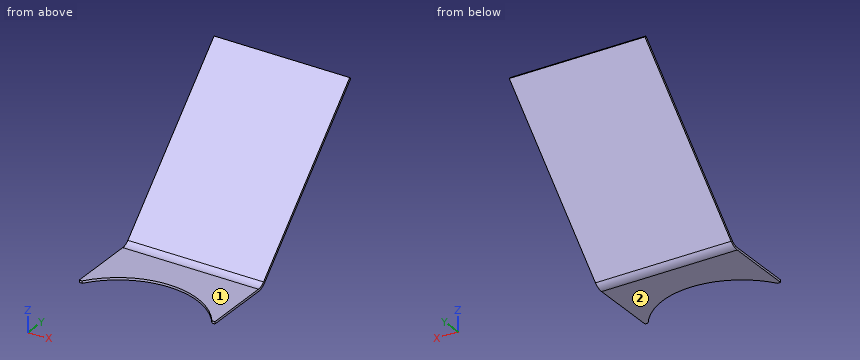
```python
from build123d import *

# Parameters (mm, degrees)
SKETCH_2_W             = 120
SKETCH_2_H             = 60
SM_BASE_FLANGE_1_DEPTH = 2
SM_EDGE_FLANGE_1_DEPTH = 120
CUT_EXTRUDE_3_REACH    = 256.546
SKETCH_3_R             = 70


# Sheet-metal steps are written as plain solids
with BuildPart() as part:
    # Sketch 2 → Базовая кромка1 (new body)
    with BuildSketch(Plane.XY):
        with Locations((60, 30)):
            Rectangle(SKETCH_2_W, SKETCH_2_H)
    extrude(amount=SM_BASE_FLANGE_1_DEPTH)

    # Ребро-кромка1 section (across the edge) → Ребро-кромка1 (add)
    with BuildSketch(Plane(origin=(120, 64.142135624, 2), x_dir=(0, -0.7071067811865438, 0.7071067811865512), z_dir=(-1, 0, 0))):
        with BuildLine():
            Line((-2, 4.142135624), (-2, 172.171572875))
            Line((-2, 172.171572875), (0, 172.171572875))
            Line((0, 172.171572875), (0, 4.142135624))
            ThreePointArc((0, 4.142135624), (0.761204675, 0.3153013), (2.928932188, -2.928932188))
            Line((2.928932188, -2.928932188), (1.514718626, -4.343145751))
            ThreePointArc((1.514718626, -4.343145751), (-1.08655439, -0.450065565), (-2, 4.142135624))
        make_face()
    extrude(amount=SM_EDGE_FLANGE_1_DEPTH)

    # Эскиз3 → Вырез-Вытянуть3 (cut, up to next)
    with BuildSketch(Plane.XY, mode=Mode.PRIVATE) as cut_extrude_3_sk1:
        with Locations((60, -40)):
            Circle(SKETCH_3_R)
    cut_extrude_3_tool1 = extrude(cut_extrude_3_sk1.sketch, amount=CUT_EXTRUDE_3_REACH, mode=Mode.PRIVATE) & part.part
    add(cut_extrude_3_tool1.solids().sort_by_distance((60, -40, 0))[0], mode=Mode.SUBTRACT)


solid = part.part
```
The model under review builds one solid part; all positions refer to its coordinate system, in mm. Face numbers are marked on the shaded views. A direction names the side the tool comes from. Coordinates: 2 decimals unless noted, no trailing zeros. Write each loop counter-clockwise with the first axis right and the second up, starting at its lowest first coordinate (ties: lowest second). Pieces come first, ordered by that corner, then holes.
1) Machinability: for the marked faces 1 and 2, which of the approach directions +Z, -Z, +X, -X, +Y, -Y give a long, thin tool a straight path to every point of the face, cutting with its end or side? Answer none if there is none.
2) We need section B-B on x = 97.5. State the section outline as (y, z) points, then the cut area to 3 significant figures.
3) Clearance check with flat-ended pins moving along their axes: pin 1 Ø6 at (x, y) = (86.5, 82) entering from +Z; pin 2 Ø4 at (x, z) = (87, 59) entering from -Y; pin 3 Ø3 at (x, y) = (93, 102.5) entering from -Z. State where each tip first meets the part, or that it passes through.
4) To check wall thickness, follow probe 1 along Z at (x, y) = (30, 48); probe 2 along Z at (x, y) = (29.5, 153); probe 3 along Y at (x, z) = (44, 106). State the ranges of each line that lie inside material, in increasing order.
5) We need section C-C on x = 18.5. State the section outline as (y, z) points.
6) We need section D-D on z = 65.5. State the section outline as (x, y) points, then the cut area to 3 significant figures.
7) We need section A-A on y = 20. State the section outline as (x, z) points.
Answer list:
1. face 1: +Z, +X, -X, -Y
1. face 2: -Z, +X, -X, +Y, -Y
2. outline: (19.11, 0) - (60, 0) arc R12 ccw to (68.49, 3.51) - (187.3, 122.33) - (185.89, 123.74) - (67.07, 4.93) arc R10 cw to (60, 2) - (19.11, 2) - close
2. area: 435 mm2
3. pin 1: stops at z = 22.86
3. pin 2: stops at y = 119.14
3. pin 3: stops at z = 36.03
4. probe 1: z = 0 to 2
4. probe 2: z = 88.03 to 90.86
4. probe 3: y = 168.14 to 170.97
5. outline: (16.37, 0) - (60, 0) arc R12 ccw to (68.49, 3.51) - (187.3, 122.33) - (185.89, 123.74) - (67.07, 4.93) arc R10 cw to (60, 2) - (16.37, 2) - close
6. outline: (0, 127.64) - (120, 127.64) - (120, 130.47) - (0, 130.47) - close
6. area: 339 mm2
7. outline: (0, 0) - (23.94, 0) - (23.94, 2) - (0, 2) - close; (96.06, 0) - (120, 0) - (120, 2) - (96.06, 2) - close
